Source: CAD feature listing. Evaluate the final solid. Frame: model axes, mm. Face numbers are marked on the shaded views. A direction names the side the tool comes from. Coordinates: 2 decimals unless noted, no trailing zeros. Write each loop counter-clockwise with the first axis right and the second up, starting at its lowest first coordinate (ties: lowest second). Pieces come first, ordered by that corner, then holes. Notation, with made-up numbers: (-0.5, 48) -> (49.5, 48) arc R20 cw to (49.5, 73) -> close; hole circle Ø7 at (34, -14.5). An arc over 180 degrees is marked (long way). One line per item, written item: value. Start each with the question number.
1. Access query for the marked faces 1 and 2. Directions: +Z, -Z, +X, -X, +Y, -Y. A direction counts if a zero-diameter tool reaches every point of the face in a straight line with its end or side. Return the directions, or none.
2. First-contact query: P1, Ø2, axis at x = -20.5, y = 26, coming from the -Z side. Flat tip, straight axial feed; report the tip coordinate or a pass-through.
3. Mould query, pull axis X, two halves, no side actions, for the marked faces 3, 4 and 5. Classes: released by +X, released by -X, zero draft, split by the parting line, or undercut.
4. Line query: line 1 (X direction, y = -22, z = 121.5); line 2 (Y direction, x = 13.5, z = 336); line 3 (Z direction, x = 25.75, y = 0). Output: solid intervals per line, ascending.
5. Section query A-A, the plane z = 310. Output: boundary loops of the cut face in (x, y), and give its area (3 significant figures).
6. Section query C-C, the plane y = 0. Output: boundary loops of the cut face in (x, z).
7. Section query B-B, the plane x = 6. Output: boundary loops of the cut face in (y, z).
8. Section query D-D, the plane z = 81. Output: boundary loops of the cut face in (x, y), and give its area (3 significant figures).
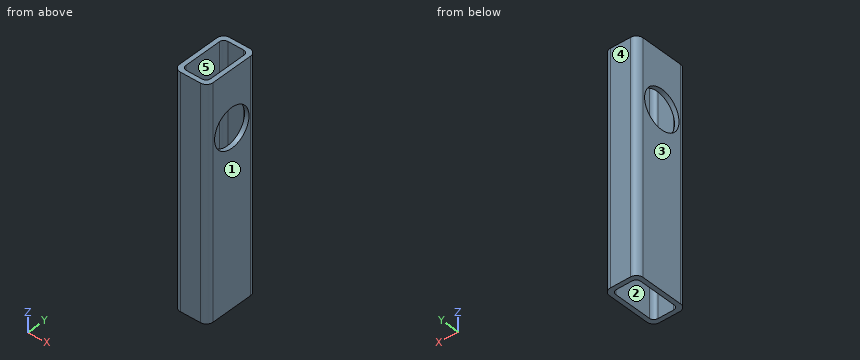
Autodesk Inventor part; units mm, degrees
ref_plane "Startebene" through (0, 0, 0) normal (0, 0, 1) x (1, 0, 0)
ref_plane "Endebene" through (0, 0, 410) normal (0, 0, 1) x (1, 0, 0)
ref_plane "YZ Plane" through (0, 0, 0) normal (1, 0, 0) x (0, 1, 0)
ref_plane "Startebene" through (0, 0, 0) normal (0, 0, 1) x (1, 0, 0)
ref_plane "Endebene" through (0, 0, 410) normal (0, 0, 1) x (1, 0, 0)
sketch "Skizze" plane through (0, 0, 0) normal (0, 0, 1) x (1, 0, 0)
  line L0 (-30, -38) -> (-30, 38)
  line L1 (-18, 50) -> (18, 50)
  line L2 (30, 38) -> (30, -38)
  line L3 (18, -50) -> (-18, -50)
  arc A0 (-30, -38) -> (-18, -50) centre (-18, -38) ccw
  arc A1 (-18, 50) -> (-30, 38) centre (-18, 38) ccw
  arc A2 (30, 38) -> (18, 50) centre (18, 38) ccw
  arc A3 (18, -50) -> (30, -38) centre (18, -38) ccw
  line L4 (-14, 42) -> (14, 42)
  line L5 (22, 34) -> (22, -34)
  line L6 (14, -42) -> (-14, -42)
  line L7 (-22, -34) -> (-22, 34)
  line L8 (0, 73.4794) -> (0, -73.4794) construction
  line L9 (-45.4794, 0) -> (45.4794, 0) construction
  arc A4 (-22, -34) -> (-14, -42) centre (-14, -34) ccw
  arc A5 (-14, 42) -> (-22, 34) centre (-14, 34) ccw
  arc A6 (22, 34) -> (14, 42) centre (14, 34) ccw
  arc A7 (14, -42) -> (22, -34) centre (14, -34) ccw
  dimension "d7" = 12
  dimension "d10" = 100
  dimension "d11" = 60
  dimension "d12" = 8
  dimension "d15" = 50
  dimension "d16" = 30
  dimension "d19" = 8
  dimension "d20" = 8
extrude "Körper" add sketch "Skizze" along normal up to surface (410 mm away) from surface at 0
sketch "Sketch3" plane through (0, 0, 0) normal (0, 0, 1) x (1, 0, 0)
  line L0 (0, 0) -> (10, 0)
ref_plane "Work Plane3" through (0, 0, 0) normal (0, -1, 0) x (1, 0, 0)
sketch "Sketch4" plane through (0, 0, 0) normal (0, -1, 0) x (1, 0, 0)
  line L0 (-2, 0) -> (12, 0)
  line L1 (-2, 410) -> (12, 410)
  dimension "d18" = 410
sketch "Skizze5" plane through (30, -38, 410) normal (1, 0, 0) x (0, 0, -1)
  line L0 (410, -12) -> (0, -12)
  line L1 (0, 76) -> (0, 0)
  point P0 (410, 38)
  point P1 (100, 38)
  dimension "d21" = 50
  dimension "d30" = 100
hole "Bohrung1" at (30, 0, 310) direction (-1, 0, 0) diameter 70 end through all
equation "\"d7\" = G_IR"
equation "\"d10\" = G_H"
equation "\"d11\" = G_W"
equation "\"d12\" = G_T"
equation "\"d15\" = 0.5 * d10"
equation "\"d16\" = 0.5 * d11"
equation "\"d19\" = G_T"
equation "\"d20\" = G_T"
equation "\"d3\" = G_L"
equation "\"G_W\" = 60"
equation "\"G_H\" = 100"
equation "\"G_T\" = 8"
equation "\"G_IR\" = 12"
equation "\"G_L\" = d18"
equation "\"G_OFFSET_START\" = 0"
equation "\"G_OFFSET_END\" = 0"
properties part number "EN 10210-2 - 90 x 50 x 5 - 400" material "Stahl, weich"
Computed values:
1. face 1: +Z, -Z, +X, +Y, -Y
1. face 2: +Z, -Z
2. P1: passes through
3. face 3: released by -X
3. face 4: zero draft
3. face 5: undercut
4. line 1: x = -30 to -22, 22 to 30
4. line 2: y = -50 to -42, 42 to 50
4. line 3: z = 0 to 275, 345 to 410
5. outline: (-30, -38) arc R12 ccw to (-18, -50) -> (18, -50) arc R12 ccw to (30, -38) -> (30, -35) -> (21.94, -35) arc R8 cw to (14, -42) -> (-14, -42) arc R8 cw to (-21.94, -35) -> (-30, -35) -> close; (-30, 35) -> (-21.94, 35) arc R8 cw to (-14, 42) -> (14, 42) arc R8 cw to (21.94, 35) -> (30, 35) -> (30, 38) arc R12 ccw to (18, 50) -> (-18, 50) arc R12 ccw to (-30, 38) -> close
5. area: 1,120 mm²
6. outline: (-30, 0) -> (-22, 0) -> (-22, 275) -> (-30, 275) -> close; (-30, 345) -> (-22, 345) -> (-22, 410) -> (-30, 410) -> close; (22, 0) -> (30, 0) -> (30, 275) -> (22, 275) -> close; (22, 345) -> (30, 345) -> (30, 410) -> (22, 410) -> close
7. outline: (-50, 0) -> (-42, 0) -> (-42, 410) -> (-50, 410) -> close; (42, 0) -> (50, 0) -> (50, 410) -> (42, 410) -> close
8. outline: (-30, -38) arc R12 ccw to (-18, -50) -> (18, -50) arc R12 ccw to (30, -38) -> (30, 38) arc R12 ccw to (18, 50) -> (-18, 50) arc R12 ccw to (-30, 38) -> close; hole (-22, -34) arc R8 ccw to (-14, -42) -> (14, -42) arc R8 ccw to (22, -34) -> (22, 34) arc R8 ccw to (14, 42) -> (-14, 42) arc R8 ccw to (-22, 34) -> close
8. area: 2,240 mm²
